Read the model definition and answer for the solid it produces. Units are mm, in the model's axes. Give positions to 0.01 mm unless a question says otherwise; leave off trailing zeros. Loops run counter-clockwise (first coordinate to the right, second up) from the corner with the lowest first, then second, coordinate; pieces in that order, holes last. Notation, with made-up numbers: M 53.5,30 L 63.5,30 A13 cw 63.5,38 Z; hole C -1.75,88 d8. An arc over 180 degrees is marked long. Return JSON: item names as keys, results as strings. Group by question number.
```python
from build123d import *

# Parameters (mm, degrees)
F1_DEPTH = 70
F2_R     = 2
F4_DEPTH = 100


with BuildPart() as f1:
    # F0 (on Top) → F1 (new body)
    with BuildSketch(Plane.XY):
        Polygon((-24.748737, -24.748737), (0, -35), (24.748737, -24.748737), (35, 0), (24.748737, 24.748737), (0, 35), (-24.748737, 24.748737), (-35, 0), align=None)
    extrude(amount=F1_DEPTH)

    # F2
    f2_edges = [f1.edges().sort_by_distance(p)[0] for p in [
        (0, -35, 35),
        (-24.748737, -24.748737, 35),
        (24.748737, -24.748737, 35),
        (35, 0, 35),
        (24.748737, 24.748737, 35),
        (0, 35, 35),
        (-24.748737, 24.748737, 35),
        (-35, 0, 35),
        (-12.374369, -29.874369, 0),
        (12.374369, -29.874369, 0),
        (29.874369, -12.374369, 0),
        (29.874369, 12.374369, 0),
        (12.374369, 29.874369, 0),
        (-12.374369, 29.874369, 0),
        (-29.874369, 12.374369, 0),
        (-29.874369, -12.374369, 0),
    ]]
    fillet(f2_edges, radius=F2_R)

    # F3 (on face) → F4 (join)
    with BuildSketch(Plane.XY.offset(70)):
        with BuildLine():
            ThreePointArc((29.874369, -12.374369), (31.714461, -6.308399), (32.335784, 0))
            ThreePointArc((32.335784, 0), (31.714461, 6.308398), (29.874369, 12.374369))
            ThreePointArc((29.874369, 12.374369), (22.864852, 22.864852), (12.374369, 29.874369))
            ThreePointArc((12.374369, 29.874369), (0, 32.335784), (-12.374368, 29.874369))
            ThreePointArc((-12.374368, 29.874369), (-22.864852, 22.864852), (-29.874369, 12.374369))
            ThreePointArc((-29.874369, 12.374369), (-32.335784, 0), (-29.874369, -12.374369))
            ThreePointArc((-29.874369, -12.374369), (-22.864852, -22.864852), (-12.374369, -29.874369))
            ThreePointArc((-12.374369, -29.874369), (0, -32.335784), (12.374368, -29.874369))
            ThreePointArc((12.374368, -29.874369), (22.864852, -22.864852), (29.874369, -12.374369))
        make_face()
    extrude(amount=F4_DEPTH)


solid = f1.part
```
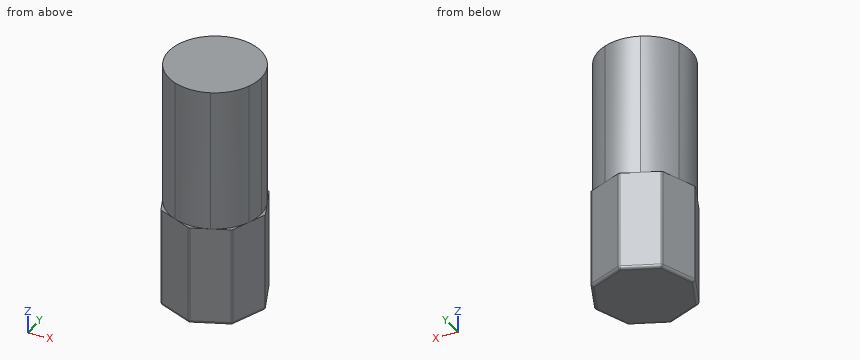
1. Straight lines are drawn through the part: line 1 along X through (y, z) = (27, 31.5); line 2 along Z through (x, y) = (-28, -12); line 3 along X through (y, z) = (-14.5, 34). For each, find the intervals that lie inside material, in ascending order.
2. Flat-ended cylindrical pins translate along their axes: P1, Ø12, axis at y = -8, z = 76.5, coming from the -X side; P2, Ø2, axis at x = -2.5, z = 152.5, coming from the -Y side; P3, Ø1.5, axis at x = -22, y = -19.5, coming from the -Z side; P4, Ø12, axis at y = -8.5, z = 44.5, coming from the -X side. Find the tip coordinate at first contact, or state that the pin passes through.
3. Find section A-A (z = 64.5). Write down the section's boundary in (x, y), and give its area (3 significant figures).
Result:
{
 "1": {"line 1": "x = -19.31 to 19.31", "line 2": "z = 0 to 170", "line 3": "x = -28.99 to 28.99"},
 "2": {"P1": "stops at x = -32.27", "P2": "stops at y = -32.3", "P3": "stops at z = 0", "P4": "stops at x = -33.96"},
 "3": {"outline": "M -34.68,-0.77 L -25.07,-23.98 A2 ccw -23.98,-25.07 L -0.77,-34.68 A2 ccw 0.77,-34.68 L 23.98,-25.07 A2 ccw 25.07,-23.98 L 34.68,-0.77 A2 ccw 34.68,0.77 L 25.07,23.98 A2 ccw 23.98,25.07 L 0.77,34.68 A2 ccw -0.77,34.68 L -23.98,25.07 A2 ccw -25.07,23.98 L -34.68,0.77 A2 ccw Z", "area": "3,460 mm2"}
}
